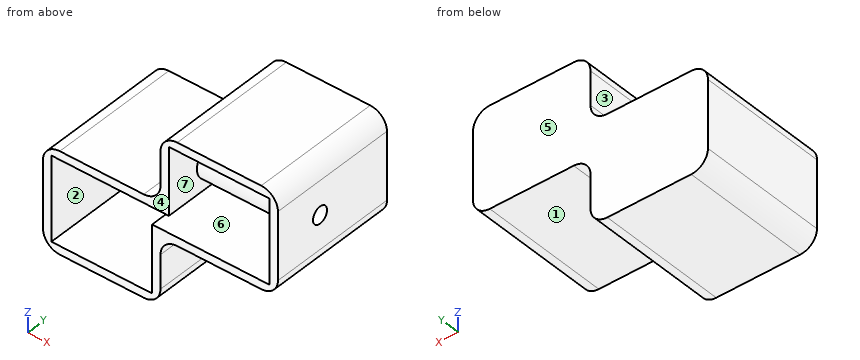
```python
from build123d import *

# Parameters (mm, degrees)
F1_DEPTH    = 38.9
F3_D        = 5
F4_T        = -2.5
F5_T1_DEPTH = 38.9
F5_T6_DEPTH = 38.9
F5_S7_R     = 2.5
F5_T8_DEPTH = 21
F5_T9_DEPTH = 63.9


# Not quite as in the source:
# - a fillet or chamfer that OpenCascade refuses, or shapes differently, is made with other operations: its cross-section is extruded or revolved along the edge and cut away or added


with BuildPart() as f1:
    # F0 (on Front) → F1 (new body)
    with BuildSketch(Plane.XZ):
        Polygon((0, 10), (0, 0), (35, 0), (35, 30), (0, 30), align=None)
        Polygon((0, -20), (0, 0), (0, 10), (-35, 10), (-35, -20), align=None)
    extrude(amount=-F1_DEPTH)

    # F3 (through all)
    with Locations(Plane.YZ.offset(35)):
        with Locations((15, 15)):
            Hole(F3_D / 2)

    # F4
    f4_openings = [f1.faces().sort_by_distance(p)[0] for p in [
        (0, 0, 5),
    ]]
    offset(amount=F4_T, openings=f4_openings, kind=Kind.INTERSECTION)

    # F5: fillet of radius 5 on 8 edges, made by hand

    # F5_s2 → F5_t1 (join)
    with BuildSketch(Plane.XZ.offset(-38.9)):
        with BuildLine():
            ThreePointArc((5, 0), (1.4644660941, -1.4644660941), (0, -5))
            Line((0, -5), (0, 0))
            Line((0, 0), (5, 0))
        make_face()
    extrude(amount=F5_T1_DEPTH)


with BuildPart() as f5_tool4:
    # F5_s5 → F5_t6 (new body)
    with BuildSketch(Plane.XZ):
        with BuildLine():
            ThreePointArc((0, 15), (-1.4644660941, 11.4644660941), (-5, 10))
            Line((-5, 10), (0, 10))
            Line((0, 10), (0, 15))
        make_face()
    extrude(amount=-F5_T6_DEPTH)

    # F5_s7 → F5_t8 (cut, symmetric)
    with BuildSketch(Plane.YZ.offset(-2.5)):
        with Locations((15, 15)):
            Circle(F5_S7_R)
    extrude(amount=F5_T8_DEPTH, both=True, mode=Mode.SUBTRACT)


with BuildPart() as f1_1:
    add(f1.part)

    # F5_t3: union F5_tool4
    add(f5_tool4.part)

    # F5_s10 → F5_t9 (cut)
    with BuildSketch(Plane.XZ.offset(-51.4)):
        with BuildLine():
            ThreePointArc((-30, 10), (-33.5355339059, 8.5355339059), (-35, 5))
            Line((-35, 5), (-35, 10))
            Line((-35, 10), (-30, 10))
        make_face()
        with BuildLine():
            ThreePointArc((-5, -20), (-1.4644660941, -18.5355339059), (0, -15))
            Line((0, -15), (0, -20))
            Line((0, -20), (-5, -20))
        make_face()
        with BuildLine():
            ThreePointArc((30, 0), (33.5355339059, 1.4644660941), (35, 5))
            Line((35, 5), (35, 0))
            Line((35, 0), (30, 0))
        make_face()
        with BuildLine():
            ThreePointArc((5, 30), (1.4644660941, 28.5355339059), (0, 25))
            Line((0, 25), (0, 30))
            Line((0, 30), (5, 30))
        make_face()
        with BuildLine():
            ThreePointArc((-35, -15), (-33.5355339059, -18.5355339059), (-30, -20))
            Line((-30, -20), (-35, -20))
            Line((-35, -20), (-35, -15))
        make_face()
        with BuildLine():
            ThreePointArc((35, 25), (33.5355339059, 28.5355339059), (30, 30))
            Line((30, 30), (35, 30))
            Line((35, 30), (35, 25))
        make_face()
    extrude(amount=F5_T9_DEPTH, mode=Mode.SUBTRACT)


solid = f1_1.part
```
The listing builds one solid part. Answer for the finished solid, in the listing's coordinates (mm). Face numbers are marked on the shaded views. A direction names the side the tool comes from. Round coordinates to 2 decimals unless told otherwise and drop trailing zeros. Order: outer loops, then holes, each group sorted by start corner. A loop starts at its lowest first (then second) coordinate and runs counter-clockwise, first axis right, second up. Notation, with made-up numbers: (75.5, 83) - (86.5, 83) arc R19 cw to (86.5, 93) - close; hole circle Ø6 at (-6.5, 34.25). An arc over 180 degrees is marked (long way). Put each result on its own line as item: value. Start each with the question number.
(1) Find section C-C (z = 19). Give the vertices of the cut face in (x, y).
(2) Straight lines are drawn through the part: probe 1 along Z at (x, y) = (24, 15); probe 2 along Z at (x, y) = (28, 29.5); probe 3 along X at (y, z) = (28, -11.5). For each, find the intervals that lie inside material, in ascending order. Write a range as from..to.
(3) Find section D-D (y = 24). Give the vertices of the cut face in (x, z).
(4) Determine the mould class of the marked faces 5, 6 and 7 for opening direction Y: released by +Y, released by -Y, zero draft, split by the parting line, or undercut.
(5) Given P1, Ø7.5, axis at x = 14, y = 19.5, coming from the -Z side; P2, Ø3, axis at y = 17, z = 20.5, coming from the -X side; P3, Ø12.5, axis at x = -19.5, y = 14.5, coming from the +Z side, each flat-ended and moving along its own axis, determine where each tip first touches the part or whether it passes through.
(6) Find section B-B (x = 1). Give the vertices of the cut face in (y, z), plus the area to 3 significant figures.
(7) For the marked faces 1, 2, 3 and 4, determine the directions among +Z, -Z, +X, -X, +Y, -Y from which every point of the face is accessible in a straight line to the end or side of a thin tool.
(8) Find section A-A (y = 15). State how many separate pieces and enclosed holes the cut face has, plus the area to 3 significant figures.
Reply:
1. outline: (0, 0) - (2.5, 0) - (2.5, 12) - (32.5, 12) - (32.5, 0) - (35, 0) - (35, 38.9) - (0, 38.9) - close; hole (2.5, 18) - (32.5, 18) - (32.5, 36.4) - (2.5, 36.4) - close
2. probe 1: 0..2.5, 10..12.5, 17.5..20, 27.5..30
2. probe 2: 0..2.5, 27.5..30
2. probe 3: -35..-32.5, -2.5..0
3. outline: (-35, -15) arc R5 ccw to (-30, -20) - (-5, -20) arc R5 ccw to (0, -15) - (0, -5) arc R5 cw to (5, 0) - (30, 0) arc R5 ccw to (35, 5) - (35, 25) arc R5 ccw to (30, 30) - (5, 30) arc R5 ccw to (0, 25) - (0, 15) arc R5 cw to (-5, 10) - (-30, 10) arc R5 ccw to (-35, 5) - close; hole (-32.5, -17.5) - (-2.5, -17.5) - (-2.5, 2.5) - (32.5, 2.5) - (32.5, 27.5) - (2.5, 27.5) - (2.5, 7.5) - (-32.5, 7.5) - close
4. face 5: released by +Y
4. face 6: zero draft
4. face 7: undercut
5. P1: z = 0
5. P2: x = 0
5. P3: z = 10
6. outline: (0, -2) - (38.9, -2) - (38.9, 28) - (0, 28) - (0, 7.5) - (36.4, 7.5) - (36.4, 2.5) - (0, 2.5) - close; hole circle Ø5 at (15, 15)
6. area: 965 mm^2
7. face 1: -Z, +X, +Y, -Y
7. face 2: -Y
7. face 3: +Z, -X, +Y, -Y
7. face 4: +Z, -Z, +X, -X, -Y
8. separate pieces: 2
8. enclosed holes: 2
8. area: 678 mm^2
